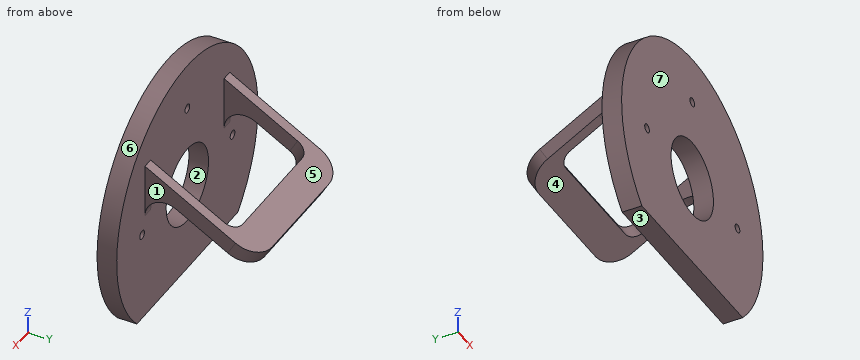
Autodesk Inventor part; units mm, degrees
ref_plane "YZ Plane" through (0, 0, 0) normal (1, 0, 0) x (0, 1, 0)
ref_plane "XZ Plane" through (0, 0, 0) normal (0, 1, 0) x (-1, 0, 0)
ref_plane "XY Plane" through (0, 0, 0) normal (0, 0, 1) x (1, 0, 0)
sketch "草图1" plane through (0, 0, 0) normal (0, 1, 0) x (-1, 0, 0)
  circle A0 centre (0, 0) radius 100
  circle A1 centre (0, 0) radius 64 construction
  point P0 (64, 0)
  point P1 (0, 64)
  point P2 (-64, 0)
  dimension "d0" = 200
  dimension "d1" = 128
extrude "拉伸1" add sketch "草图1" against normal blind 15
hole "孔1" at (-64, 0, 0) at (0, 0, 64) at (64, 0, 0) direction (0, -1, 0) diameter 6.647 end through all
hole "孔2" at (0, 0, 0) direction (0, -1, 0) diameter 60 end through all
sketch "草图2" plane through (0, 0, 0) normal (1, 0, 0) x (0, 1, 0)
  line L0 (0, 55) -> (86.6025, 5)
  line L1 (86.6025, 5) -> (80.6025, -5.3923)
  line L2 (80.6025, -5.3923) -> (24, 27.2872)
  line L3 (0, 27.5) -> (0, 0)
  line L4 (0, 0) -> (0, 13.4308)
  arc A0 (24, 27.2872) -> (0, 13.4308) centre (16, 13.4308) ccw
  line L5 (0, -100) -> (0, 100)
  line L6 (0, 55) -> (0, 13.4308)
  point P0 (0, 13.4308)
  dimension "d19" = 55
  dimension "d20" = 100
  dimension "d22" = 12
  dimension "d23" = 0
  dimension "d24" = 16
extrude "拉伸2" add sketch "草图2" along normal mid plane 120
sketch "草图3" plane through (-60, 86.6025, 5) normal (0, 0.5, 0.8660254) x (1, 0, 0)
  line L0 (120, -100) -> (0, -100)
  line L1 (48.0104, -100) -> (71.9896, -100)
  line L2 (120, -100) -> (0, -100)
  line L3 (120, -100) -> (112, -100)
  line L4 (112, -100) -> (112, -35)
  line L5 (0, -100) -> (0, -79.2154)
  line L6 (0, -100) -> (8, -100)
  line L7 (8, -100) -> (8, -35)
  line L8 (18, -25) -> (102, -25)
  line L9 (112, -100) -> (8, -100)
  arc A0 (18, -25) -> (8, -35) centre (18, -35) ccw
  arc A1 (112, -35) -> (102, -25) centre (102, -35) ccw
  point P0 (60, -72.5)
  point P1 (112, -25)
  point P2 (8, -25)
  dimension "d27" = 8
  dimension "d28" = 75
  dimension "d29" = 8
  dimension "d30" = 75
  dimension "d31" = 10
extrude "拉伸3" cut sketch "草图3" against normal up to surface surface through (0, 0, 0) normal (0, 1, 0)
fillet "圆角1" radius 20 2 edges at (60, 83.6025, -0.1962) (-60, 83.6025, -0.1962)
sketch "草图4" plane through (0, 0, 0) normal (0, 1, 0) x (1, 0, 0)
  circle A0 centre (0, 0) radius 100
  line L0 (0, 0) -> (0, 70)
  line L1 (0, 70) -> (-92.5065, 70)
  line L2 (-92.5065, 70) -> (-88.0231, 170.2178)
  line L3 (-88.0231, 170.2178) -> (67.3235, 163.2683)
  line L4 (67.3235, 163.2683) -> (102.3961, 70)
  line L5 (0, 70) -> (102.3961, 70)
  point P0 (71.4143, 70)
  point P1 (-71.4143, 70)
  dimension "d35" = 70
extrude "拉伸4" cut sketch "草图4" against normal through all contours L5 L1 A0 picked at (-44.3165, 72.9417)
properties part number "2"
Can you work these out from the model? Positions are in its coordinate system, mm. Face numbers are marked on the shaded views. A direction names the side the tool comes from. Give positions to 0.01 mm unless a question says otherwise; leave off trailing zeros. Loops run counter-clockwise (first coordinate to the right, second up) from the corner with the lowest first, then second, coordinate; pieces in that order, holes last. Notation, with made-up numbers: (-2, 61) - (20, 61) arc R18 cw to (20, 81) - close; hole circle Ø1 at (26.25, 69). An arc over 180 degrees is marked (long way). One line per item, written item: value.
(1) If we section it at B-B, the plane y = -6: List the corners of the cut face in (x, z) for me, plus the area to 3 significant figures.
Verdict:
outline: (-71.41, -70) - (71.41, -70) arc R100 ccw (long way) to start; hole circle Ø6.65 at (-64, 0); hole circle Ø60 at (0, 0); hole circle Ø6.65 at (0, 64); hole circle Ø6.65 at (64, 0)
area: 25,500 mm^2
(2) I'm going to push flat-ended pins straight in: pin 1 (8 mm diameter, centred on x = -62, y = 58.5, fed in from +Z) (3 decimals); pin 2 (4 mm diameter, centred on x = -64, z = 0, fed in from -Y); pin 3 (3 mm diameter, centred on x = -43, z = 66.5, fed in from +Y); pin 4 (4 mm diameter, centred on x = -55, y = 21.5, fed in from -Z). Where does each tip first touch, or does it pass through?
Verdict:
pin 1: z = 23.225
pin 2: through
pin 3: y = 0
pin 4: z = 27.56
(3) If we mould it in two halves opening along Y, with no side actions, what happens to the marked faces 4, 5, 6 and 7? For each: released by +Y, released by -Y, zero draft, split by the parting line, or undercut.
Verdict:
face 4: undercut
face 5: released by +Y
face 6: zero draft
face 7: released by -Y
(4) If we section it at D-D, the plane z = 64: List the corners of the cut face in (x, y) for me.
Verdict:
outline: (-76.84, -15) - (-3.32, -15) - (-3.32, 0) - (-76.84, 0) - close; (3.32, -15) - (76.84, -15) - (76.84, 0) - (3.32, 0) - close
(5) If we section it at C-C, the plane x = 64: List the corners of the cut face in (y, z) for me, plus the area to 3 significant figures.
Verdict:
outline: (-15, -70) - (0, -70) - (0, -3.32) - (-15, -3.32) - close; (-15, 3.32) - (0, 3.32) - (0, 76.84) - (-15, 76.84) - close
area: 2,100 mm^2
(6) On a 3-axis mill with a long thin cutter (end or side, diameter ignored), from which of +Z, -Z, +X, -X, +Y, -Y can I reach the whole of each face in a straight line? I mean the marked faces 1, 2 and 3. Say none if no direction works.
Verdict:
face 1: +Z, -Z, +X, +Y
face 2: -Y
face 3: -Z, +X, -X, +Y, -Y
(7) If we section it at A-A, the plane x = 0: List the corners of the cut face in (y, z) for me, plus the area to 3 significant figures.
Verdict:
outline: (-15, -70) - (0, -70) - (0, -30) - (-15, -30) - close; (-15, 30) - (0, 30) - (0, 60.68) - (-15, 60.68) - close; (-15, 67.32) - (0, 67.32) - (0, 100) - (-15, 100) - close; (58.95, 7.11) - (80.6, -5.39) - (86.6, 5) - (64.95, 17.5) - close
area: 1,850 mm^2
(8) I need wall thicknesses on line 1 along Z through (x, y) = (0, -8); line 2 along X through (y, z) = (-6, 0); line 3 along X through (y, z) = (20.5, 40). Which ranges of each line are inside material? Lowest first, please.
Verdict:
line 1: -70 to -30, 30 to 60.68, 67.32 to 100
line 2: -100 to -67.32, -60.68 to -30, 30 to 60.68, 67.32 to 100
line 3: -60 to -52, 52 to 60
